Could you check a few things on this drawing? It's one solid part, dimensions in mm from its lowest x, y, z. Give positions to 0.01 mm unless a question says otherwise; leave off trailing zeros. Loops run counter-clockwise (first coordinate to the right, second up) from the corner with the lowest first, then second, coordinate; pieces in that order, holes last. Notation, with made-up numbers: M -31.75,46.25 L -18.75,46.25 A20 cw -18.75,64.25 Z; hole C 33,-20 d6. An arc over 180 degrees is marked long. Answer as CSV lines item,"result". Start each with the question number.
Item 1: I want a section at D-D on z = 19. List the corners of the cut face in (x, y) for me.
Item 2: If I drill on line 1 along X through (y, z) = (5.2, 60); line 2 along X through (y, z) = (4.05, 14.5), over which ranges is the centre line in solid material (lowest first)? Write a range as from..to.
Item 3: I want a section at A-A on x = 61. List the corners of the cut face in (y, z) for me.
Item 4: Will these pins go through, and if not, where does the flat tip stop? P1, Ø3, axis at y = 2.5, z = 91.5, coming from the -X side; P2, Ø1.8, axis at x = 30.5, y = 2, coming from the -Z side; P3, Ø4.5, axis at x = 46.5, z = 52.76, coming from the -Y side; P4, Ø1.8, axis at x = 107, y = 4.5, coming from the +Z side.
Item 5: I want a section at B-B on y = 2.5. List the corners of the cut face in (x, z) for me, plus the area to 3 significant figures.
Item 6: I want a section at C-C on x = 7. List the corners of the cut face in (y, z) for me.
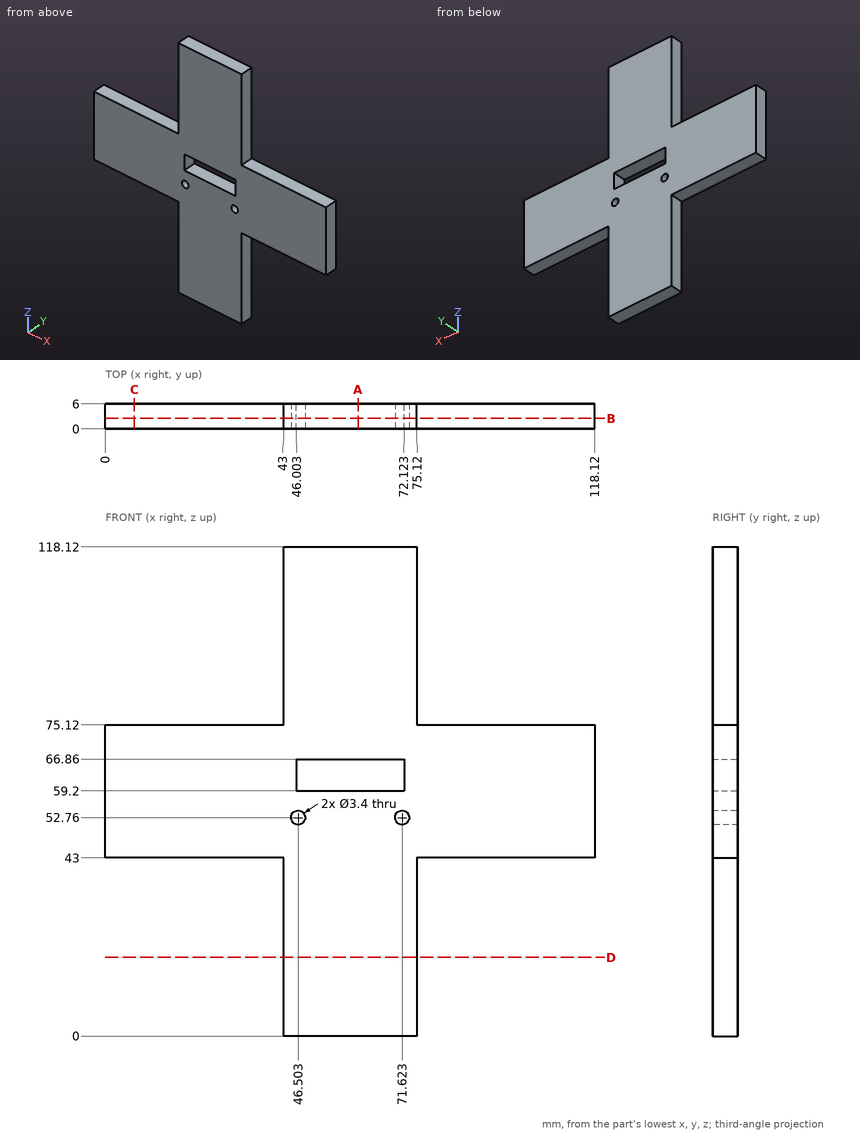
Result:
1,outline,"M 43,0 L 75.12,0 L 75.12,6 L 43,6 Z"
2,line 1,"0..46, 72.12..118.12"
2,line 2,"43..75.12"
3,outline,"M 0,0 L 6,0 L 6,59.2 L 0,59.2 Z; M 0,66.86 L 6,66.86 L 6,118.12 L 0,118.12 Z"
4,P1,"x = 43"
4,P2,"z = 43"
4,P3,"y = 0"
4,P4,"z = 75.12"
5,outline,"M 0,43 L 43,43 L 43,0 L 75.12,0 L 75.12,43 L 118.12,43 L 118.12,75.12 L 75.12,75.12 L 75.12,118.12 L 43,118.12 L 43,75.12 L 0,75.12 Z; hole C 46.5,52.76 d3.4; hole M 46,59.2 L 72.12,59.2 L 72.12,66.86 L 46,66.86 Z; hole C 71.62,52.76 d3.4"
5,area,"6,340 mm^2"
6,outline,"M 0,43 L 6,43 L 6,75.12 L 0,75.12 Z"
